For this review, take the finished solid that the model builds, in its own axes (mm). A direction names the side the tool comes from. Give positions to 0.01 mm unless a question says otherwise; leave off trailing zeros. Order: outer loops, then holes, each group sorted by start corner. A loop starts at its lowest first (then second) coordinate and runs counter-clockwise, first axis right, second up. Notation, with made-up numbers: (-30.75, 51.5) - (25.25, 51.5) arc R15 ccw to (25.25, 64.5) - close; hole circle Ø3 at (-6, -35.75). An arc over 180 degrees is marked (long way). Put each result on its own line as item: value. Start each with the question number.
```python
from build123d import *

# Parameters (mm, degrees)
SKETCH1_W           = 48
SKETCH1_H           = 26
SKETCH1_R           = 5.25
BOSS_EXTRUDE1_DEPTH = 55
CUT_EXTRUDE1_REACH  = 67.399
SKETCH2_R           = 2.75
SKETCH3_R           = 4.5
CUT_EXTRUDE2_DEPTH  = 4.5
CUT_EXTRUDE3_REACH  = 63.4
SKETCH4_R           = 1.75
SKETCH5_R           = 3
CUT_EXTRUDE4_DEPTH  = 15
SKETCH6_R           = 11.25
CUT_EXTRUDE5_DEPTH  = 30
BOSS_EXTRUDE3_DEPTH = 55
SKETCH10_W          = 42.5
SKETCH10_H          = 42.5
SKETCH10_R          = 1.65
SKETCH10_R_2        = 11.5
BOSS_EXTRUDE4_DEPTH = 7
CHAMFER1_SIZE       = 2
SKETCH11_W          = 42.5
SKETCH11_H          = 42.5
SKETCH11_R          = 11.5
SKETCH11_R_2        = 1.75
BOSS_EXTRUDE5_DEPTH = 3
FILLET2_R           = 20
CHAMFER2_SIZE       = 2
BOSS_EXTRUDE6_DEPTH = 58
SKETCH13_R          = 2.25
CUT_EXTRUDE6_DEPTH  = 126.672192628
SKETCH14_R          = 3.75
CUT_EXTRUDE7_DEPTH  = 5
SKETCH15_R          = 2.25
CUT_EXTRUDE8_DEPTH  = 8
SKETCH16_R          = 3.75
CUT_EXTRUDE9_DEPTH  = 1
SKETCH17_R          = 3
CUT_EXTRUDE10_DEPTH = 2


with BuildPart() as part:
    # Sketch1 → Boss-Extrude1 (new body)
    with BuildSketch(Plane(origin=(0, 0, 0), x_dir=(1, 0, 0), z_dir=(0, 1, 0))):
        Rectangle(SKETCH1_W, SKETCH1_H)
        with Locations(Location((0, 0, 0), (0, 0, 270))):
            Circle(SKETCH1_R, mode=Mode.SUBTRACT)
    extrude(amount=BOSS_EXTRUDE1_DEPTH)

    # Sketch2 → Cut-Extrude1 (cut, up to next)
    with BuildSketch(Plane.XY.offset(13), mode=Mode.PRIVATE) as cut_extrude1_sk1:
        with Locations((-16, 45.5)):
            Circle(SKETCH2_R)
    cut_extrude1_tool1 = extrude(cut_extrude1_sk1.sketch, amount=-CUT_EXTRUDE1_REACH, mode=Mode.PRIVATE) & part.part
    # Sketch2 → Cut-Extrude1 (cut, up to next)
    with BuildSketch(Plane.XY.offset(13), mode=Mode.PRIVATE) as cut_extrude1_sk2:
        with Locations((16, 45.5)):
            Circle(SKETCH2_R)
    cut_extrude1_tool2 = extrude(cut_extrude1_sk2.sketch, amount=-CUT_EXTRUDE1_REACH, mode=Mode.PRIVATE) & part.part
    # Sketch2 → Cut-Extrude1 (cut, up to next)
    with BuildSketch(Plane.XY.offset(13), mode=Mode.PRIVATE) as cut_extrude1_sk3:
        with Locations((16, 9.5)):
            Circle(SKETCH2_R)
    cut_extrude1_tool3 = extrude(cut_extrude1_sk3.sketch, amount=-CUT_EXTRUDE1_REACH, mode=Mode.PRIVATE) & part.part
    # Sketch2 → Cut-Extrude1 (cut, up to next)
    with BuildSketch(Plane.XY.offset(13), mode=Mode.PRIVATE) as cut_extrude1_sk4:
        with Locations((-16, 9.5)):
            Circle(SKETCH2_R)
    cut_extrude1_tool4 = extrude(cut_extrude1_sk4.sketch, amount=-CUT_EXTRUDE1_REACH, mode=Mode.PRIVATE) & part.part
    add(cut_extrude1_tool1.solids().sort_by_distance((-16, 45.5, 13))[0], mode=Mode.SUBTRACT)
    add(cut_extrude1_tool2.solids().sort_by_distance((16, 45.5, 13))[0], mode=Mode.SUBTRACT)
    add(cut_extrude1_tool3.solids().sort_by_distance((16, 9.5, 13))[0], mode=Mode.SUBTRACT)
    add(cut_extrude1_tool4.solids().sort_by_distance((-16, 9.5, 13))[0], mode=Mode.SUBTRACT)

    # Sketch3 → Cut-Extrude2 (cut)
    with BuildSketch(Plane.XY.offset(13)):
        with Locations((-16, 45.5)):
            Circle(SKETCH3_R)
        with Locations(Location((16, 45.5, 0), (0, 0, 180))):
            Circle(SKETCH3_R)
        with Locations((16, 9.5)):
            Circle(SKETCH3_R)
        with Locations(Location((-16, 9.5, 0), (0, 0, 180))):
            Circle(SKETCH3_R)
    extrude(amount=-CUT_EXTRUDE2_DEPTH, mode=Mode.SUBTRACT)

    # Sketch4 → Cut-Extrude3 (cut, up to next)
    with BuildSketch(Plane(origin=(0, 55, 0), x_dir=(1, 0, 0), z_dir=(0, 1, 0)), mode=Mode.PRIVATE) as cut_extrude3_sk1:
        with Locations(Location((0, 8, 0), (0, 0, 270))):
            Circle(SKETCH4_R)
    cut_extrude3_tool1 = extrude(cut_extrude3_sk1.sketch, amount=-CUT_EXTRUDE3_REACH, mode=Mode.PRIVATE) & part.part
    # Sketch4 → Cut-Extrude3 (cut, up to next)
    with BuildSketch(Plane(origin=(0, 55, 0), x_dir=(1, 0, 0), z_dir=(0, 1, 0)), mode=Mode.PRIVATE) as cut_extrude3_sk2:
        with Locations(Location((8, 0, 0), (0, 0, 270))):
            Circle(SKETCH4_R)
    cut_extrude3_tool2 = extrude(cut_extrude3_sk2.sketch, amount=-CUT_EXTRUDE3_REACH, mode=Mode.PRIVATE) & part.part
    # Sketch4 → Cut-Extrude3 (cut, up to next)
    with BuildSketch(Plane(origin=(0, 55, 0), x_dir=(1, 0, 0), z_dir=(0, 1, 0)), mode=Mode.PRIVATE) as cut_extrude3_sk3:
        with Locations(Location((0, -8, 0), (0, 0, 270))):
            Circle(SKETCH4_R)
    cut_extrude3_tool3 = extrude(cut_extrude3_sk3.sketch, amount=-CUT_EXTRUDE3_REACH, mode=Mode.PRIVATE) & part.part
    # Sketch4 → Cut-Extrude3 (cut, up to next)
    with BuildSketch(Plane(origin=(0, 55, 0), x_dir=(1, 0, 0), z_dir=(0, 1, 0)), mode=Mode.PRIVATE) as cut_extrude3_sk4:
        with Locations(Location((-8, 0, 0), (0, 0, 270))):
            Circle(SKETCH4_R)
    cut_extrude3_tool4 = extrude(cut_extrude3_sk4.sketch, amount=-CUT_EXTRUDE3_REACH, mode=Mode.PRIVATE) & part.part
    add(cut_extrude3_tool1.solids().sort_by_distance((0, 55, -8))[0], mode=Mode.SUBTRACT)
    add(cut_extrude3_tool2.solids().sort_by_distance((8, 55, 0))[0], mode=Mode.SUBTRACT)
    add(cut_extrude3_tool3.solids().sort_by_distance((0, 55, 8))[0], mode=Mode.SUBTRACT)
    add(cut_extrude3_tool4.solids().sort_by_distance((-8, 55, 0))[0], mode=Mode.SUBTRACT)

    # Sketch5 → Cut-Extrude4 (cut)
    with BuildSketch(Plane(origin=(0, 55, 0), x_dir=(1, 0, 0), z_dir=(0, 1, 0))):
        with Locations((0, 8)):
            Circle(SKETCH5_R)
        with Locations((8, 0)):
            Circle(SKETCH5_R)
        with Locations((0, -8)):
            Circle(SKETCH5_R)
        with Locations((-8, 0)):
            Circle(SKETCH5_R)
    extrude(amount=-CUT_EXTRUDE4_DEPTH, mode=Mode.SUBTRACT)

    # Sketch6 → Cut-Extrude5 (cut)
    with BuildSketch(Plane.XZ):
        with Locations(Location((0, 0, 0), (0, 0, 270))):
            Circle(SKETCH6_R)
    extrude(amount=-CUT_EXTRUDE5_DEPTH, mode=Mode.SUBTRACT)

    # Sketch9 → Boss-Extrude3 (add)
    with BuildSketch(Plane(origin=(0, 55, 0), x_dir=(1, 0, 0), z_dir=(0, 1, 0))):
        Polygon((-24, -13), (-29, -13), (-29, 57), (29, 57), (29, -13), (24, -13), (24, 47), (-24, 47), align=None)
    extrude(amount=-BOSS_EXTRUDE3_DEPTH)

    # Sketch10 → Boss-Extrude4 (add)
    with BuildSketch(Plane(origin=(0, 0, -57), x_dir=(-1, 0, 0), z_dir=(0, 0, -1))):
        with Locations((-50.25, 33.75)):
            Rectangle(SKETCH10_W, SKETCH10_H)
        with Locations((-65.75, 49.25)):
            Circle(SKETCH10_R, mode=Mode.SUBTRACT)
        with Locations(Location((-34.75, 49.25, 0), (0, 0, 180))):
            Circle(SKETCH10_R, mode=Mode.SUBTRACT)
        with Locations((-34.75, 18.25)):
            Circle(SKETCH10_R, mode=Mode.SUBTRACT)
        with Locations(Location((-65.75, 18.25, 0), (0, 0, 180))):
            Circle(SKETCH10_R, mode=Mode.SUBTRACT)
        with Locations((-50.25, 33.75)):
            Circle(SKETCH10_R_2, mode=Mode.SUBTRACT)
    extrude(amount=-BOSS_EXTRUDE4_DEPTH)

    # Chamfer1
    chamfer1_edges = [part.edges().sort_by_distance(p)[0] for p in [
        (71.5, 12.5, -53.5),
        (71.5, 55, -53.5),
    ]]
    chamfer(chamfer1_edges, length=CHAMFER1_SIZE)

    # Sketch11 → Boss-Extrude5 (add)
    with BuildSketch(Plane(origin=(0, 55, 0), x_dir=(1, 0, 0), z_dir=(0, 1, 0))):
        with Locations((50.25, -9.25)):
            Rectangle(SKETCH11_W, SKETCH11_H)
        with Locations(Location((50.25, -9.25, 0), (0, 0, 270))):
            Circle(SKETCH11_R, mode=Mode.SUBTRACT)
        with Locations(Location((34.75, 6.25, 0), (0, 0, 270))):
            Circle(SKETCH11_R_2, mode=Mode.SUBTRACT)
        with Locations(Location((65.75, 6.25, 0), (0, 0, 90))):
            Circle(SKETCH11_R_2, mode=Mode.SUBTRACT)
        with Locations(Location((65.75, -24.75, 0), (0, 0, 270))):
            Circle(SKETCH11_R_2, mode=Mode.SUBTRACT)
        with Locations(Location((34.75, -24.75, 0), (0, 0, 90))):
            Circle(SKETCH11_R_2, mode=Mode.SUBTRACT)
    extrude(amount=-BOSS_EXTRUDE5_DEPTH)

    # Fillet2
    # the kernel refuses this fillet: 20 mm, written as the material it adds along each edge
    with BuildSketch(Plane(origin=(29, 55, 13), x_dir=(-1, 0, 0), z_dir=(0, -1, 0))) as fillet2_piece_1:
        with BuildLine():
            CenterArc((19.843134833, -20), FILLET2_R, 90, 82.819244219)
            Line((0, -17.5), (0, 0))
            Line((0, 0), (19.843134833, 0))
        make_face()
    extrude(amount=3)

    # Chamfer2
    chamfer2_edges = [part.edges().sort_by_distance(p)[0] for p in [
        (71.5, 53.5, -12),
        (71.5, 53.5, 30.5),
    ]]
    chamfer(chamfer2_edges, length=CHAMFER2_SIZE)

    # Sketch12 → Boss-Extrude6 (add)
    with BuildSketch(Plane(origin=(29, 0, 0), x_dir=(0, 0, -1), z_dir=(1, 0, 0))):
        Polygon((57, 0), (85.3, 18.75), (85.3, 23.75), (85.3, 43.75), (77.3, 43.75), (77.3, 23.75), (57, 23.75), align=None)
    extrude(amount=-BOSS_EXTRUDE6_DEPTH)

    # Sketch13 → Cut-Extrude6 (cut, through all)
    with BuildSketch(Plane(origin=(0, 0, -57), x_dir=(-1, 0, 0), z_dir=(0, 0, -1))):
        with Locations((15, 33.75)):
            Circle(SKETCH13_R)
        with Locations((-15, 33.75)):
            Circle(SKETCH13_R)
    extrude(amount=-CUT_EXTRUDE6_DEPTH, mode=Mode.SUBTRACT)

    # Sketch14 → Cut-Extrude7 (cut)
    with BuildSketch(Plane.XY.offset(-47)):
        with Locations((-15, 33.75)):
            Circle(SKETCH14_R)
        with Locations((15, 33.75)):
            Circle(SKETCH14_R)
    extrude(amount=-CUT_EXTRUDE7_DEPTH, mode=Mode.SUBTRACT)

    # Sketch15 → Cut-Extrude8 (cut)
    with BuildSketch(Plane(origin=(0, 0, -85.3), x_dir=(-1, 0, 0), z_dir=(0, 0, -1))):
        with Locations((-14, 33.75)):
            Circle(SKETCH15_R)
        Polygon((29, 43.75), (1, 43.75), (1, 23.75), (1, 11.75), (29, 11.75), (29, 23.75), align=None)
    extrude(amount=-CUT_EXTRUDE8_DEPTH, mode=Mode.SUBTRACT)

    # Sketch16 → Cut-Extrude9 (cut)
    with BuildSketch(Plane(origin=(0, 0, -85.3), x_dir=(-1, 0, 0), z_dir=(0, 0, -1))):
        with Locations((-14, 33.75)):
            Circle(SKETCH16_R)
    extrude(amount=-CUT_EXTRUDE9_DEPTH, mode=Mode.SUBTRACT)

    # Sketch17 → Cut-Extrude10 (cut)
    with BuildSketch(Plane(origin=(0, 0, -57), x_dir=(-1, 0, 0), z_dir=(0, 0, -1))):
        with Locations((-65.75, 49.25)):
            Circle(SKETCH17_R)
        with Locations(Location((-34.75, 49.25, 0), (0, 0, 180))):
            Circle(SKETCH17_R)
        with Locations((-34.75, 18.25)):
            Circle(SKETCH17_R)
        with Locations(Location((-65.75, 18.25, 0), (0, 0, 180))):
            Circle(SKETCH17_R)
    extrude(amount=-CUT_EXTRUDE10_DEPTH, mode=Mode.SUBTRACT)


solid = part.part
```
1. Wall thickness on line 1 (Z direction, x = 16, y = 40); line 2 (Z direction, x = -8, y = 43); line 3 (X direction, y = 20.5, z = -17.5): over which ranges is each line inside the solid? List them lowest first. Write a range as from..to.
2. Add section D-D, the plane x = 27. Give the boundary of the cut face in (y, z), then the cut area to 3 significant figures.
3. Tool access review of faces 5 (the face through (15.642, 48.227, -2.099)), 6 (the face through (-1, 29, -81)), 7 (the face through (-11, 48, 0)): name each direction out of +Z, -Z, +X, -X, +Y, -Y from which nothing blocks a thin tool from reaching the whole face with its end or side.
4. The part is to be moulded in two halves that separate along Z. For faces 1 (the face through (64, 48, -55)), 2 (the face through (-13, 32, -52)), 3 (the face through (14.81, 30.09, -84.81)), 4 (the face through (-15.81, 30.09, -49.46)), say which applies: released by +Z, released by -Z, zero draft, split by the parting line, or undercut.
5. Clearance check with flat-ended pins moving along their axes: pin 1 (5 mm diameter, centred on x = -15.5, y = 19.5, fed in from -Z); pin 2 (9.5 mm diameter, centred on x = 65.75, y = 49.25, fed in from -Z); pin 3 (4 mm diameter, centred on x = -18, y = 26.5, fed in from +Z). State where each tip first meets the part, or that it passes through.
6. Add section C-C, the plane z = 17.5. Give the boundary of the cut face in (x, y).
7. Add section B-B, the plane x = 43.5. Give the boundary of the cut face in (y, z).
8. Add section A-A, the plane y = 26.5. Give the boundary of the cut face in (x, z), then the cut area to 3 significant figures.
Found:
1. line 1: z = -85.3..-77.3, -57..-47, -13..13
1. line 2: z = -57..-47, -13..-3, 3..13
1. line 3: x = -29..-24, 24..29
2. outline: (0, -57) - (18.75, -85.3) - (43.75, -85.3) - (43.75, -77.3) - (23.75, -77.3) - (23.75, -57) - (55, -57) - (55, 23.97) - (52, 23.97) - (52, 13) - (0, 13) - close
2. area: 4,450 mm^2
3. face 5: +Z
3. face 6: -Z, -X, +Y, -Y
3. face 7: +Y
4. face 1: released by -Z
4. face 2: undercut
4. face 3: zero draft
4. face 4: undercut
5. pin 1: stops at z = -77.3
5. pin 2: stops at z = -57
5. pin 3: stops at z = 13
6. outline: (21.8, 52) - (42.24, 52) - (42.24, 55) - (21.8, 55) - close; (58.26, 52) - (71.5, 52) - (71.5, 55) - (58.26, 55) - close
7. outline: (12.5, -57) - (24.44, -57) - (24.44, -50) - (12.5, -50) - close; (43.06, -57) - (55, -57) - (55, -50) - (43.06, -50) - close; (52, -12) - (55, -12) - (55, -0.06) - (52, -0.06) - close; (52, 18.56) - (55, 18.56) - (55, 30.5) - (52, 30.5) - close
8. outline: (-29, -57) - (41.32, -57) - (41.32, -50) - (29, -50) - (29, 13) - (-29, 13) - close; (-1, -85.3) - (29, -85.3) - (29, -77.3) - (-1, -77.3) - close; (59.18, -57) - (71.5, -57) - (71.5, -50) - (59.18, -50) - close; hole (-24, -47) - (24, -47) - (24, -13) - (-24, -13) - close; hole circle Ø22.5 at (0, 0)
8. area: 2,440 mm^2
